from build123d import *

# Parameters (mm, degrees)
F0_W     = 76.2
F0_H     = 91.7677478655
F1_DEPTH = 7.366
F2_W     = 118.1442663074
F2_H     = 12.3756490648
F3_DEPTH = 34.798
F4_DEPTH = 40.894
F5_R     = 6.35
F6_DEPTH = 25.4


with BuildPart() as f1:
    # F0 (on Right) → F1 (new body)
    with BuildSketch(Plane.YZ):
        with Locations((2.8780587018, 1.5829317272)):
            Rectangle(F0_W, F0_H)
    extrude(amount=F1_DEPTH)

    # F2 (on Front) → F3 (join)
    with BuildSketch(Plane.XZ):
        with Locations((59.0721331537, -49.7903954238)):
            Rectangle(F2_W, F2_H)
    extrude(amount=F3_DEPTH)

    # F2 (on Front) → F4 (join)
    with BuildSketch(Plane.XZ):
        with Locations((59.0721331537, -49.7903954238)):
            Rectangle(F2_W, F2_H)
    extrude(amount=-F4_DEPTH)

    # F5 (on face) → F6 (cut)
    with BuildSketch(Plane(origin=(0, 0, -55.9782199562), x_dir=(1, 0, 0), z_dir=(0, 0, -1))):
        with Locations((20.9336709231, -23.0455552376)):
            Circle(F5_R)
        with Locations((20.9336709231, 17.1015182538)):
            Circle(F5_R)
    extrude(amount=-F6_DEPTH, mode=Mode.SUBTRACT)


solid = f1.part
Build history of the part. All positions in model axes, mm. A direction names the side the tool comes from. Round coordinates to 2 decimals unless told otherwise and drop trailing zeros. Write each loop counter-clockwise with the first axis right and the second up, starting at its lowest first coordinate (ties: lowest second). Pieces come first, ordered by that corner, then holes. Notation, with made-up numbers: (61.25, 21.5) - (66.25, 21.5) arc R30 cw to (66.25, 53.5) - close; hole circle Ø7 at (17, 22). An arc over 180 degrees is marked (long way). One line per question, with ' | ' between items.
1. Mould opens along X. For faces 3 (the face through (58, -34.798, -50)), 4 (the face through (118.144, 3, -50)), 5 (the face through (0, 2, -5)), 6 (the face through (26.8, 25.48, -49.88)) say: released by +X, released by -X, zero draft, split by the parting line, or undercut.
Results are:
face 3: zero draft | face 4: released by +X | face 5: released by -X | face 6: undercut
2. Band-saw the part on D-D, the plane y = -28. Write the cut outline in (x, z), and give its area (3 significant figures).
Results are:
outline: (0, -55.98) - (118.14, -55.98) - (118.14, -43.6) - (7.37, -43.6) - (7.37, 47.47) - (0, 47.47) - close | area: 2,130 mm^2
3. Band-saw the part on A-A, the plane x = 24.5. Write the cut outline in (y, z).
Results are:
outline: (-34.8, -55.98) - (-22.36, -55.98) - (-22.36, -43.6) - (-34.8, -43.6) - close; (-11.85, -55.98) - (17.79, -55.98) - (17.79, -43.6) - (-11.85, -43.6) - close; (28.3, -55.98) - (40.89, -55.98) - (40.89, -43.6) - (28.3, -43.6) - close
4. Band-saw the part on C-C, the plane z = -46. Write the cut outline in (x, y), and give its area (3 significant figures).
Results are:
outline: (0, -34.8) - (118.14, -34.8) - (118.14, 40.89) - (0, 40.89) - close; hole circle Ø12.7 at (20.93, -17.1); hole circle Ø12.7 at (20.93, 23.05) | area: 8,690 mm^2
5. Tool access for faces 1 (the face through (24.347, -22.456, -49.877)), 2 (the face through (62, 3, -43.603)): list every direction of +Z, -Z, +X, -X, +Y, -Y with a clear straight run to the whole face (end or side of a thin tool).
Results are:
face 1: +Z, -Z | face 2: +Z, +X, +Y, -Y
6. Band-saw the part on B-B, the plane y = -13.5. Write the cut outline in (x, z).
Results are:
outline: (0, -55.98) - (15.7, -55.98) - (15.7, -43.6) - (7.37, -43.6) - (7.37, 47.47) - (0, 47.47) - close; (26.16, -55.98) - (118.14, -55.98) - (118.14, -43.6) - (26.16, -43.6) - close
7. Drill centre lines: line 1 along Z through (x, y) = (95, 18.5); line 2 along X through (y, z) = (1.5, 12.5). Where is each one in solid material? Low to high. Write a range as from..to.
Results are:
line 1: -55.98..-43.6 | line 2: 0..7.37
8. Drop flat-ended pins along their axis: pin 1 Ø3 at (y, z) = (23, -6) entering from +X; pin 2 Ø10 at (x, z) = (60, -48.5) entering from -Y; pin 3 Ø16.5 at (x, y) = (20.93, 23.05) entering from +Z. Give the stop position or say it passes through.
Results are:
pin 1: x = 7.37 | pin 2: y = -34.8 | pin 3: z = -43.6
